Autodesk Inventor part; units mm, degrees
ref_plane "YZ Plane" through (0, 0, 0) normal (1, 0, 0) x (0, 1, 0)
ref_plane "XZ Plane" through (0, 0, 0) normal (0, 1, 0) x (-1, 0, 0)
ref_plane "XY Plane" through (0, 0, 0) normal (0, 0, 1) x (1, 0, 0)
sketch "Sketch1" plane through (0, 0, 0) normal (0, 0, 1) x (1, 0, 0)
  line L0 (-212.5, -82.5) -> (212.5, -82.5)
  line L1 (212.5, -82.5) -> (212.5, 82.5)
  line L2 (212.5, 82.5) -> (-212.5, 82.5)
  line L3 (-212.5, 82.5) -> (-212.5, -82.5)
  line L4 (-212.5, -82.5) -> (212.5, 82.5) construction
  line L5 (212.5, -82.5) -> (-212.5, 82.5) construction
  line L6 (0, 118.3995) -> (0, -118.3995) construction
  circle A0 centre (0, 71.5) radius 2.25
  circle A1 centre (-192.5, 71.5) radius 2.25
  line L7 (-300.3995, 0) -> (300.3995, 0)
  circle A2 centre (192.5, 71.5) radius 2.25
  circle A3 centre (0, -71.5) radius 2.25 construction
  circle A4 centre (-192.5, -71.5) radius 2.25
  circle A5 centre (192.5, -71.5) radius 2.25
  line L8 (-194.25, 0.5) -> (-194.25, -40.0844) construction
  circle A6 centre (0, -79.5) radius 2.25
  point P0 (0, 0)
  dimension "d0" = 425
  dimension "d1" = 165
  dimension "d2" = 4.5
  dimension "d3" = 71.5
  dimension "d4" = 192.5
  dimension "d5" = 4.5
  dimension "d6" = 71.5
  dimension "d12" = 72
  dimension "d14" = 194.25
  dimension "d24" = 8
  dimension "d25" = 4.5
extrude "Extrusion1" add sketch "Sketch1" along normal blind 3
fillet "Fillet1" radius 10 4 edges at (-212.5, -82.5, 1.5) (-212.5, 82.5, 1.5) (212.5, -82.5, 1.5) (212.5, 82.5, 1.5)
sketch "Sketch3" plane through (0, 0, 3) normal (0, 0, 1) x (1, 0, 0)
  line L0 (17.5, 82.5) -> (167.5, 82.5)
  line L1 (167.5, 82.5) -> (167.5, 63.5)
  line L2 (167.5, 63.5) -> (17.5, 63.5)
  line L3 (17.5, 63.5) -> (17.5, 82.5)
  line L4 (202.5, 82.5) -> (-202.5, 82.5)
  line L5 (212.5, -72.5) -> (212.5, 72.5)
  point P0 (0, 0)
  dimension "d18" = 45
  dimension "d19" = 150
  dimension "d20" = 19
extrude "Extrusion2" cut sketch "Sketch3" against normal blind 3
fillet "Fillet2" radius 2 4 edges at (17.5, 63.5, 1.5) (17.5, 82.5, 1.5) (167.5, 82.5, 1.5) (167.5, 63.5, 1.5)
sketch "Sketch6" plane through (0, 0, 3) normal (0, 0, 1) x (1, 0, 0)
  line L0 (0, 117.5) -> (0, -127.5)
  line L1 (-202.5, -82.5) -> (202.5, -82.5)
  line L2 (-202.5, -82.5) -> (202.5, -82.5)
  line L3 (-44, -82.5) -> (-34, -92.5)
  line L4 (-34, -92.5) -> (0, -92.5)
  line L5 (44, -82.5) -> (34, -92.5)
  line L6 (34, -92.5) -> (0, -92.5)
  point P0 (0, 0)
  dimension "d26" = 45
  dimension "d27" = 10
extrude "Extrusion3" add sketch "Sketch6" against normal up to surface (3 mm away)
fillet "Fillet3" radius 10 4 edges at (-44, -82.5, 1.5) (-34, -92.5, 1.5) (34, -92.5, 1.5) (44, -82.5, 1.5)
sketch "Sketch7" plane through (0, 0, 3) normal (0, 0, 1) x (1, 0, 0)
  circle A0 centre (192.5, 71.5) radius 2.25
  circle A1 centre (-192.5, 71.5) radius 2.25
  circle A2 centre (0, 71.5) radius 2.25
  circle A3 centre (-192.5, -71.5) radius 2.25
  circle A4 centre (192.5, -71.5) radius 2.25
  circle A5 centre (0, -79.5) radius 2.25
  arc A6 (29.8579, -92.5) -> (36.9289, -89.5711) centre (29.8579, -82.5) ccw
  line L0 (36.9289, -89.5711) -> (41.0711, -85.4289)
  arc A7 (48.1421, -82.5) -> (41.0711, -85.4289) centre (48.1421, -92.5) ccw
  line L1 (48.1421, -82.5) -> (202.5, -82.5)
  arc A8 (202.5, -82.5) -> (212.5, -72.5) centre (202.5, -72.5) ccw
  line L2 (212.5, -72.5) -> (212.5, 72.5)
  arc A9 (212.5, 72.5) -> (202.5, 82.5) centre (202.5, 72.5) ccw
  line L3 (202.5, 82.5) -> (169.5, 82.5)
  arc A10 (169.5, 82.5) -> (167.5, 80.5) centre (169.5, 80.5) ccw
  line L4 (167.5, 80.5) -> (167.5, 65.5)
  arc A11 (165.5, 63.5) -> (167.5, 65.5) centre (165.5, 65.5) ccw
  line L5 (165.5, 63.5) -> (19.5, 63.5)
  arc A12 (17.5, 65.5) -> (19.5, 63.5) centre (19.5, 65.5) ccw
  line L6 (17.5, 65.5) -> (17.5, 80.5)
  arc A13 (17.5, 80.5) -> (15.5, 82.5) centre (15.5, 80.5) ccw
  line L7 (15.5, 82.5) -> (-202.5, 82.5)
  arc A14 (-202.5, 82.5) -> (-212.5, 72.5) centre (-202.5, 72.5) ccw
  line L8 (-212.5, 72.5) -> (-212.5, -72.5)
  arc A15 (-212.5, -72.5) -> (-202.5, -82.5) centre (-202.5, -72.5) ccw
  line L9 (-202.5, -82.5) -> (-48.1421, -82.5)
  arc A16 (-41.0711, -85.4289) -> (-48.1421, -82.5) centre (-48.1421, -92.5) ccw
  line L10 (-41.0711, -85.4289) -> (-36.9289, -89.5711)
  arc A17 (-36.9289, -89.5711) -> (-29.8579, -92.5) centre (-29.8579, -82.5) ccw
  line L11 (-29.8579, -92.5) -> (29.8579, -92.5)
  point P0 (0, 0)
equation "\"d5\" = d2"
equation "\"d6\" = d3"
equation "\"d25\" = d5"
properties part number "KeyBoardHolder"
Verification items for the finished model (mm, model axes). Round coordinates to 2 decimals unless told otherwise and drop trailing zeros. Write each loop counter-clockwise with the first axis right and the second up, starting at its lowest first coordinate (ties: lowest second). Pieces come first, ordered by that corner, then holes. Notation, with made-up numbers: (-34.75, 50.25) - (-23.75, 50.25) arc R28 ccw to (-23.75, 89.25) - close; hole circle Ø3 at (-26, 16). An arc over 180 degrees is marked (long way). Answer as a JSON object with one key per item and string values. Group by question number.
Q1. Section check C-C, the plane x = 186. Enter the section's corners in (y, z), plus the area to 3 significant figures.
Q2. Go/stop test with flat-tipped pins: pin 1 Ø1.5 at (y, z) = (76, 1.5) entering from -X; pin 2 Ø1 at (x, z) = (83.5, 2) entering from -Y; pin 3 Ø2.5 at (x, y) = (0, -79.5) entering from -Z; pin 4 Ø1.5 at (x, z) = (80.5, 2) entering from +Y. Record where each tip stops, or that it passes through.
Q3. Section check A-A, the plane z = 1.05. Give the number of separate pieces and of enclosed holes in the cut face, plus the area to 3 significant figures.
Q4. Thickness scan on line 1 (Y direction, x = 192.5, z = 1.8); line 2 (Y direction, x = 0, z = 0.8); line 3 (Y direction, x = 189.5, z = 0.35). Record the ranges inside material, lowest first.
Q5. Section check B-B, the plane x = 53. Enter the section's corners in (y, z).
Found:
{
 "1": {"outline": "(-82.5, 0) - (82.5, 0) - (82.5, 3) - (-82.5, 3) - close", "area": "495 mm^2"},
 "2": {"pin 1": "stops at x = -212.11", "pin 2": "stops at y = -82.5", "pin 3": "passes through", "pin 4": "stops at y = 63.5"},
 "3": {"separate pieces": "1", "enclosed holes": "6", "area": "67,900 mm^2"},
 "4": {"line 1": "y = -82.5 to -73.75, -69.25 to 69.25, 73.75 to 82.5", "line 2": "y = -92.5 to -81.75, -77.25 to 69.25, 73.75 to 82.5", "line 3": "y = -82.5 to 82.5"},
 "5": {"outline": "(-82.5, 0) - (63.5, 0) - (63.5, 3) - (-82.5, 3) - close"}
}
